Design review of the part built by this model. Coordinates are the model's own, in mm. A direction names the side the tool comes from. Give positions to 0.01 mm unless a question says otherwise; leave off trailing zeros. Order: outer loops, then holes, each group sorted by start corner. A loop starts at its lowest first (then second) coordinate and runs counter-clockwise, first axis right, second up. Notation, with made-up numbers: M 68,87 L 120,87 A18 ccw 120,112 Z; hole C 14.25,-38 d3. An arc over 180 degrees is marked long. Answer as a JSON object with one key per item and string values.
from build123d import *

# Parameters (mm, degrees)
SKETCH_1_W          = 42
SKETCH_1_H          = 42
EXTRUDE_1_DEPTH     = 48
SKETCH_2_R          = 11
EXTRUDE_2_DEPTH     = 2
SKETCH_3_R          = 1.5
CUT_EXTRUDE_1_DEPTH = 78.640195775
SKETCH_4_R          = 2.5
EXTRUDE_3_DEPTH     = 22
CUT_EXTRUDE_START   = -18
CUT_EXTRUDE_2_DEPTH = 18


with BuildPart() as part:
    # 草图1 → 凸台-拉伸1 (new body)
    with BuildSketch(Plane(origin=(0, 0, 0), x_dir=(1, 0, 0), z_dir=(0, 1, 0))):
        with Locations((21, 21)):
            Rectangle(SKETCH_1_W, SKETCH_1_H)
    extrude(amount=EXTRUDE_1_DEPTH)

    # 草图2 → 凸台-拉伸2 (add)
    with BuildSketch(Plane(origin=(0, 48, 0), x_dir=(1, 0, 0), z_dir=(0, 1, 0))):
        with Locations(Location((21, 21, 0), (0, 0, 270))):
            Circle(SKETCH_2_R)
    extrude(amount=EXTRUDE_2_DEPTH)

    # 草图3 → 切除-拉伸1 (cut, through all)
    with BuildSketch(Plane.XZ):
        with Locations(Location((36.5, -5.5, 0), (0, 0, 270))):
            Circle(SKETCH_3_R)
        with Locations(Location((5.5, -5.5, 0), (0, 0, 270))):
            Circle(SKETCH_3_R)
        with Locations(Location((5.5, -36.5, 0), (0, 0, 270))):
            Circle(SKETCH_3_R)
        with Locations(Location((36.5, -36.5, 0), (0, 0, 270))):
            Circle(SKETCH_3_R)
    extrude(amount=-CUT_EXTRUDE_1_DEPTH, mode=Mode.SUBTRACT)

    # 草图4 → 凸台-拉伸3 (add)
    with BuildSketch(Plane(origin=(0, 50, 0), x_dir=(1, 0, 0), z_dir=(0, 1, 0))):
        with Locations(Location((21, 21, 0), (0, 0, 270))):
            Circle(SKETCH_4_R)
    extrude(amount=EXTRUDE_3_DEPTH)

    # 草图5 → 切除-拉伸2 (cut)
    with BuildSketch(Plane(origin=(0, 72, 0), x_dir=(1, 0, 0), z_dir=(0, 1, 0)).offset(CUT_EXTRUDE_START)):
        with BuildLine():
            Line((22, 23.291287847), (22, 21))
            Line((22, 21), (22, 18.708712153))
            ThreePointArc((22, 18.708712153), (23.091650066, 19.630693606), (23.5, 21))
            ThreePointArc((23.5, 21), (23.091650066, 22.369306394), (22, 23.291287847))
        make_face()
    extrude(amount=CUT_EXTRUDE_2_DEPTH, mode=Mode.SUBTRACT)


solid = part.part
(1) We need section A-A (z = -36.5). Write out the cut boundary in (x, y), plus the area to 3 significant figures.
Checked values:
{"outline": "M 0,0 L 4,0 L 4,48 L 0,48 Z; M 7,0 L 35,0 L 35,48 L 7,48 Z; M 38,0 L 42,0 L 42,48 L 38,48 Z", "area": "1,730 mm^2"}
(2) We need section B-B (y = 25.5). Write out the cut boundary in (x, z), plus the area to 3 significant figures.
Checked values:
{"outline": "M 0,-42 L 42,-42 L 42,0 L 0,0 Z; hole C 5.5,-36.5 d3; hole C 5.5,-5.5 d3; hole C 36.5,-36.5 d3; hole C 36.5,-5.5 d3", "area": "1,740 mm^2"}
(3) Tool access review of faces 5 (the flat face through (23, 54, -21)), 6 (the flat face through (21, 72, -21)), 7 (the cylindrical face through (11.241, 48.986, -15.924)): name each direction out of +Z, -Z, +X, -X, +Y, -Y from which nothing blocks a thin tool from reaching the whole face with its end or side.
Checked values:
{"face 5": "+Z, -Z, +X, +Y", "face 6": "+Z, -Z, +X, -X, +Y", "face 7": "+Y"}
(4) We need section D-D (x = 21). Write out the cut boundary in (y, z), plus the area to 3 significant figures.
Checked values:
{"outline": "M 0,-42 L 48,-42 L 48,-32 L 50,-32 L 50,-23.5 L 72,-23.5 L 72,-18.5 L 50,-18.5 L 50,-10 L 48,-10 L 48,0 L 0,0 Z", "area": "2,170 mm^2"}
(5) Insertion check: pin 1 (3.5 mm diameter, centred on x = 36.5, z = -5.5, fed in from +Y); pin 2 (1.4 mm diameter, centred on y = 59, z = -21.5, fed in from +X); pin 3 (1.5 mm diameter, centred on x = 13, z = -16, fed in from +Y). Each pin has a flat end and moves straight along its axis. Give the tip position at first contact, or say it passes through.
Checked values:
{"pin 1": "stops at y = 48", "pin 2": "stops at x = 22", "pin 3": "stops at y = 50"}
(6) To check wall thickness, follow L1, parallel to X at y = 31.5, z = -36.5; L2, parallel to Z at x = 36, y = 29; L3, parallel to Y at x = 9, z = -17. State the ranges of each line that lie inside material, in increasing order. Write a range as from..to.
Checked values:
{"L1": "x = 0..4, 7..35, 38..42", "L2": "z = -42..-37.91, -35.09..-6.91, -4.09..0", "L3": "y = 0..48"}
(7) Draft analysis for pull direction Z (two halves, no side actions). For faces 1 (the cylindrical face through (4.6, 23.7, -35.3)), 2 (the flat face through (30, 48, -12)), 3 (the cylindrical face through (18.56, 60.85, -21.54)), 4 (the flat face through (21, 24, -42)), state which applies: +Z half, -Z half, draft (parallel to the pull), parting line (faces both ways), or undercut.
Checked values:
{"face 1": "undercut", "face 2": "draft", "face 3": "parting line", "face 4": "-Z half"}
(8) We need section C-C (x = 5.5). Write out the cut boundary in (y, z), plus the area to 3 significant figures.
Checked values:
{"outline": "M 0,-42 L 48,-42 L 48,-38 L 0,-38 Z; M 0,-35 L 48,-35 L 48,-7 L 0,-7 Z; M 0,-4 L 48,-4 L 48,0 L 0,0 Z", "area": "1,730 mm^2"}
